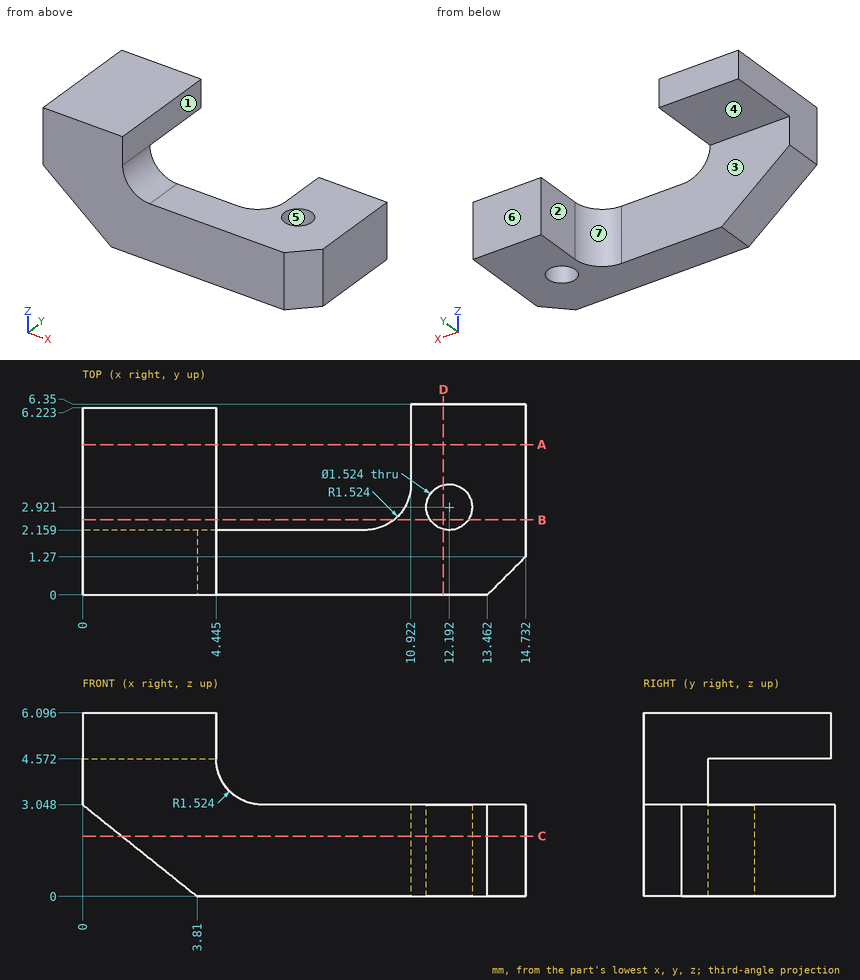
Input: dimensioned drawing with shaded views. Units: mm. Origin: part minimum x, y, z. A direction names the side the tool comes from. Coordinates: 2 decimals unless noted, no trailing zeros. Loops run counter-clockwise (first coordinate to the right, second up) from the corner with the lowest first, then second, coordinate; pieces in that order, holes last. Notation, with made-up numbers: (25, 85) -> (55, 85) arc R29 ccw to (55, 112) -> close; hole circle Ø1 at (1.25, -2.5). An arc over 180 degrees is marked (long way). One line per item, written item: value. Start each with the question number.
Q1. Section query D-D, the plane x = 12. Return the cut outline in (y, z).
Q2. Contact query for flat-ended pins moving along their axis: P1, Ø3.5, axis at x = 1, y = 5, coming from the -Z side; P2, Ø2, axis at y = 5.5, z = 1, coming from the -X side; P3, Ø1.2, axis at x = 2.5, z = 5.5, coming from the +Y side. Output: stop coordinate, or through.
Q3. Mould query, pull axis X, two halves, no side actions, for the marked faces 5, 6 and 7. Classes: pulls with the +X half, pulls with the -X half, needs draft (parallel to the pull), parting line crosses it, or undercut.
Q4. Line query: line 1 along Z through (x, y) = (4.25, 2.5); line 2 along Z through (x, y) = (11.5, 1.75); line 3 along Y through (x, z) = (2, 4.25). Output: solid intervals per line, ascending.
Q5. Set-up query: the marked faces 1, 2, 3 and 4. Return all of +Z, -Z, +X, -X, +Y, -Y with unobstructed straight access to the full face (end or side cutting, diameter ignored); none if empty.
Q6. Section query A-A, the plane y = 5. Return the cut outline in (x, z) (3 decimals).
Q7. Section query C-C, the plane z = 2. Return the cut outline in (x, y).
Q8. Section query B-B, the plane y = 2.5. Return the cut outline in (x, z) (3 decimals).
Results:
1. outline: (0, 0) -> (2.18, 0) -> (2.18, 3.05) -> (0, 3.05) -> close; (3.66, 0) -> (6.35, 0) -> (6.35, 3.05) -> (3.66, 3.05) -> close
2. P1: z = 4.57
2. P2: x = 10.92
2. P3: y = 6.22
3. face 5: undercut
3. face 6: needs draft
3. face 7: pulls with the -X half
4. line 1: 4.57 to 6.1
4. line 2: 0 to 3.05
4. line 3: 0 to 2.16
5. face 1: +Z, +X, +Y, -Y
5. face 2: +Z, -Z, -X, +Y
5. face 3: -Z, -X, +Y
5. face 4: -Z, +X, -X, +Y
6. outline: (0, 4.572) -> (4.445, 4.572) -> (4.445, 6.096) -> (0, 6.096) -> close; (10.922, 0) -> (14.732, 0) -> (14.732, 3.048) -> (10.922, 3.048) -> close
7. outline: (1.31, 0) -> (13.46, 0) -> (14.73, 1.27) -> (14.73, 6.35) -> (10.92, 6.35) -> (10.92, 3.68) arc R1.52 cw to (9.4, 2.16) -> (1.31, 2.16) -> close; hole circle Ø1.52 at (12.19, 2.92)
8. outline: (0, 4.572) -> (4.445, 4.572) -> (4.445, 6.096) -> (0, 6.096) -> close; (10.359, 0) -> (11.557, 0) -> (11.557, 3.048) -> (10.359, 3.048) -> close; (12.827, 0) -> (14.732, 0) -> (14.732, 3.048) -> (12.827, 3.048) -> close
